Read the model definition and answer for the solid it produces. Units are mm, in the model's axes. A direction names the side the tool comes from. Round coordinates to 2 decimals unless told otherwise and drop trailing zeros. Order: outer loops, then holes, each group sorted by start corner. A loop starts at its lowest first (then second) coordinate and runs counter-clockwise, first axis right, second up. Notation, with made-up numbers: (29.5, -14.5) -> (53.5, -14.5) arc R31 ccw to (53.5, 15.5) -> close; hole circle Ø8 at (-34.75, -15). An arc over 180 degrees is marked (long way). Answer as a JSON object with one key per item and string values. Group by question number.
Item 1: Given P1, Ø1, axis at y = -4.5, z = -44, coming from the -X side; P2, Ø8, axis at x = -34, y = -0.5, coming from the -Z side; P3, Ø12, axis at y = 14, z = -52, coming from the +X side, each flat-ended and moving along its own axis, determine where each tip first touches the part or whether it passes through.
Item 2: Section B-B, the plane y = -6 is taken. Write down the section's boundary in (x, z) (3 decimals).
Item 3: Section D-D, the plane z = 58 is taken. Write down the section's boundary in (x, y) (3 decimals).
Item 4: The mould has two halves that part along Y. Classify faces 1 (the flat face through (-58, 16.905, 0)), 2 (the conical face through (-62.363, 13.251, -6.233)), 3 (the cylindrical face through (-43.554, 19.455, -36.256)): pulls with the +Y half, pulls with the -Y half, needs draft (parallel to the pull), parting line crosses it, or undercut.
Item 5: Section C-C, the plane x = -40 is taken. Write down the section's boundary in (y, z) (3 decimals).
Item 6: For faces 4 (the flat face through (-64.051, 5.576, 2.926)), 5 (the flat face through (15, 7.62, 15)), 6 (the cylindrical face through (-54.57, 20.77, -25.18)), determine the directions among +Z, -Z, +X, -X, +Y, -Y from which every point of the face is accessible in a straight line to the end or side of a thin tool.
Item 7: Consider probe 1 along X at (y, z) = (13.3, 0); probe 2 along X at (y, z) = (-2.5, 0) (3 decimals); probe 3 along X at (y, z) = (5.55, 0) (3 decimals). Determine where each line is inside the solid, lowest interval first. Write a range as from..to.
Item 8: Section A-A, the plane x = 0 is taken. Write down the section's boundary in (y, z) (3 decimals), plus the area to 3 significant figures.
from build123d import *

# Parameters (mm, degrees)
GEAR_START                      = -10
SKETCH1_R                       = 10.16
GEAR_SLOT_DEPTH                 = 10
CIRPATTERN1_COUNT               = 2
CIRPATTERN1_ANGLE               = 10
CIRPATTERN1_THE_OTHER_WAY_COUNT = 2
CIRPATTERN1_THE_OTHER_WAY_ANGLE = 10
GAS_MANIFOLD_DEPTH              = 7.62


with BuildPart() as part:
    # Sketch9 → Revolve1 (revolve)
    with BuildSketch(Plane.XY, mode=Mode.PRIVATE) as revolve1_sk:
        Polygon((-10.16, 10.16), (-10.16, 24.525), (-67.5, 24.525), (-67.5, -13.575), (-63.375, -13.575), (-63.375, 10.795), (-53.825, 10.795), (-53.825, 5.08), (-46, 5.08), (-46, 6.35), (-36, 6.35), (-36, 7.62), (-21, 7.62), (-21, 10.16), align=None)
    revolve(revolve1_sk.sketch.rotate(Axis((0, 18.1216542, 0), (0, -1, 0)), 270), axis=Axis((0, 18.1216542, 0), (0, -1, 0)))

    # Sketch1 → Gear Slot (cut)
    with BuildSketch(Plane(origin=(0, 24.525, 0), x_dir=(1, 0, 0), z_dir=(0, 1, 0)).offset(GEAR_START)):
        with BuildLine():
            ThreePointArc((-60.123839141, -30.681818182), (15.778004595, -65.630058441), (67.5, 0))
            ThreePointArc((67.5, 0), (15.778004595, 65.630058441), (-60.123839141, 30.681818182))
            ThreePointArc((-60.123839141, 30.681818182), (-43.307976674, 36.134044285), (-37.85575057, 19.318181818))
            ThreePointArc((-37.85575057, 19.318181818), (-42.5, 0), (-37.85575057, -19.318181818))
            ThreePointArc((-37.85575057, -19.318181818), (-43.307976674, -36.134044285), (-60.123839141, -30.681818182))
        make_face()
        with Locations(Location((0, 0, 0), (0, 0, 270))):
            Circle(SKETCH1_R, mode=Mode.SUBTRACT)
    extrude(amount=GEAR_SLOT_DEPTH, mode=Mode.SUBTRACT)

    # Sketch5 one side → Orifice (revolve, cut)
    with BuildSketch(Plane(origin=(-60, 0, 0), x_dir=(0, 0, -1), z_dir=(1, 0, 0)), mode=Mode.PRIVATE) as orifice_sk:
        Polygon((-9.77813806, 16.364061196), (-7.26937996, 3.457619634), (-2.759272111, 5.65734621), (-10.553511101, 21.637904353), (-12.005063486, 20.929934951), align=None)
    orifice = revolve(orifice_sk.sketch.rotate(Axis((-60, 5.65734621, 2.759272111), (0, 0.8987940462991696, 0.43837114678907213)), 180), axis=Axis((-60, 5.65734621, 2.759272111), (0, 0.8987940462991696, 0.43837114678907213)), mode=Mode.SUBTRACT)

    # CirPattern1: Orifice ×2 about axis
    cirpattern1_axis = Axis((0, 17.78, 0), (0, -1, 0))
    for i in range(1, CIRPATTERN1_COUNT):
        add(orifice.rotate(cirpattern1_axis, i * CIRPATTERN1_ANGLE / (CIRPATTERN1_COUNT - 1)), mode=Mode.SUBTRACT)

    # CirPattern1 the other way: Orifice ×2 about axis
    cirpattern1_the_other_way_axis = Axis((0, 17.78, 0), (0, 1, 0))
    for i in range(1, CIRPATTERN1_THE_OTHER_WAY_COUNT):
        add(orifice.rotate(cirpattern1_the_other_way_axis, i * CIRPATTERN1_THE_OTHER_WAY_ANGLE / (CIRPATTERN1_THE_OTHER_WAY_COUNT - 1)), mode=Mode.SUBTRACT)

    # Sketch10 → Gas Manifold (cut)
    with BuildSketch(Plane(origin=(0, 24.525, 0), x_dir=(1, 0, 0), z_dir=(0, 1, 0))):
        with BuildLine():
            ThreePointArc((-51.683094143, -18.811107883), (-55, 0), (-51.683094143, 18.811107883))
            ThreePointArc((-51.683094143, 18.811107883), (-54.671456531, 25.219671703), (-61.080020351, 22.231309316))
            ThreePointArc((-61.080020351, 22.231309316), (-65, 0), (-61.080020351, -22.231309316))
            ThreePointArc((-61.080020351, -22.231309316), (-54.671456531, -25.219671703), (-51.683094143, -18.811107883))
        make_face()
    extrude(amount=-GAS_MANIFOLD_DEPTH, mode=Mode.SUBTRACT)


solid = part.part
Values found:
{
 "1": {"P1": "x = -51.61", "P2": "z = -60.47", "P3": "x = 49.4"},
 "2": {"outline": "circle Ø135 at (0, 0); hole circle Ø126.75 at (0, 0)"},
 "3": {"outline": "(-34.529, -13.575) -> (-25.542, -13.575) -> (-25.542, 10.795) -> (25.542, 10.795) -> (25.542, -13.575) -> (34.529, -13.575) -> (34.529, 14.525) -> (-34.529, 14.525) -> close"},
 "4": {"face 1": "pulls with the +Y half", "face 2": "undercut", "face 3": "needs draft"},
 "5": {"outline": "(-13.575, -54.371) -> (14.525, -54.371) -> (14.525, -33.685) -> (24.525, -33.685) -> (24.525, -14.361) -> (14.525, -14.361) -> (14.525, 14.361) -> (24.525, 14.361) -> (24.525, 33.685) -> (14.525, 33.685) -> (14.525, 54.371) -> (-13.575, 54.371) -> (-13.575, 49.157) -> (10.795, 49.157) -> (10.795, 36.016) -> (5.08, 36.016) -> (5.08, 22.716) -> (6.35, 22.716) -> (6.35, -22.716) -> (5.08, -22.716) -> (5.08, -36.016) -> (10.795, -36.016) -> (10.795, -49.157) -> (-13.575, -49.157) -> close"},
 "6": {"face 4": "none", "face 5": "-Y", "face 6": "+Y"},
 "7": {"probe 1": "-67.5..-10.16, 10.16..67.5", "probe 2": "-67.5..-63.375, 63.375..67.5", "probe 3": "-67.5..-63.375, -53.825..-46, 46..53.825, 63.375..67.5"},
 "8": {"outline": "(-13.575, -67.5) -> (14.525, -67.5) -> (14.525, -10.16) -> (10.16, -10.16) -> (10.16, -21) -> (7.62, -21) -> (7.62, -36) -> (6.35, -36) -> (6.35, -46) -> (5.08, -46) -> (5.08, -53.825) -> (10.795, -53.825) -> (10.795, -63.375) -> (-13.575, -63.375) -> close; (-13.575, 63.375) -> (10.795, 63.375) -> (10.795, 53.825) -> (5.08, 53.825) -> (5.08, 46) -> (6.35, 46) -> (6.35, 36) -> (7.62, 36) -> (7.62, 21) -> (10.16, 21) -> (10.16, 10.16) -> (14.525, 10.16) -> (14.525, 67.5) -> (-13.575, 67.5) -> close", "area": "916 mm2"}
}
